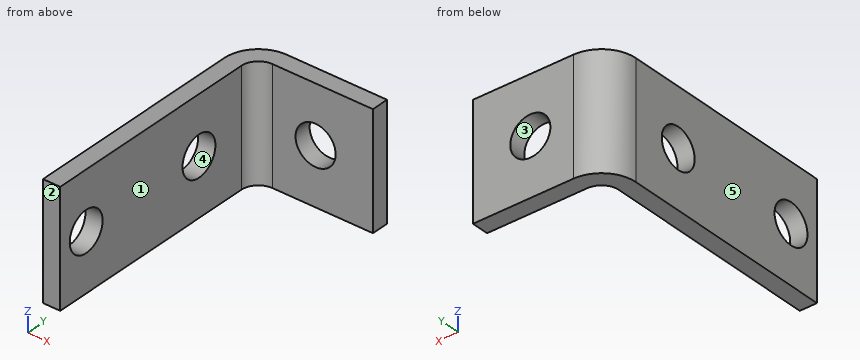
from build123d import *

# Parameters (mm, degrees)
BASE_FLANGE1_DEPTH             = 40
CUT_EXTRUDE1_DEPTH             = 109.350745652
F_14_0_14_DIAMETER_HOLE1_D     = 14
F_14_0_14_DIAMETER_HOLE1_DEPTH = 47
F_14_0_14_DIAMETER_HOLE2_D     = 14


# Sheet-metal steps are written as plain solids
with BuildPart() as part:
    # Sketch7 → Base-Flange1 (new body)
    with BuildSketch(Plane.XY):
        with BuildLine():
            Line((0, 0), (47, 0))
            Line((47, 0), (47, 89.055511246))
            Line((47, 89.055511246), (12, 89.055511246))
            ThreePointArc((12, 89.055511246), (3.514718626, 85.54079262), (0, 77.055511246))
            Line((0, 77.055511246), (0, 0))
        make_face()
    extrude(amount=-BASE_FLANGE1_DEPTH)

    # Sketch10 → Cut-Extrude1 (cut, through all)
    with BuildSketch(Plane(origin=(0, 0, -40), x_dir=(-1, 0, 0), z_dir=(0, 0, -1))):
        with BuildLine():
            Line((-12, 83.055511246), (-47, 83.055511246))
            Line((-47, 83.055511246), (-47, 0))
            Line((-47, 0), (-6, 0))
            Line((-6, 0), (-6, 77.055511246))
            ThreePointArc((-6, 77.055511246), (-7.757359313, 81.298151933), (-12, 83.055511246))
        make_face()
    extrude(amount=-CUT_EXTRUDE1_DEPTH, mode=Mode.SUBTRACT)

    # Ø14.0 (14) Diameter Hole1
    with Locations(Plane.ZY):
        with Locations((-20, 59.055511246), (-20, 11.055511246)):
            Hole(F_14_0_14_DIAMETER_HOLE1_D / 2, depth=F_14_0_14_DIAMETER_HOLE1_DEPTH)

    # Ø14.0 (14) Diameter Hole2 (through all)
    with Locations(Plane(origin=(0, 83.055511246, 0), x_dir=(-1, 0, 0), z_dir=(0, -1, 0))):
        with Locations((-27, 20)):
            Hole(F_14_0_14_DIAMETER_HOLE2_D / 2)


solid = part.part
Geometry: final body of the model. Coordinates: model frame, mm. Face numbers are marked on the shaded views. A direction names the side the tool comes from. Coordinates: 2 decimals unless noted, no trailing zeros. Order: outer loops, then holes, each group sorted by start corner. A loop starts at its lowest first (then second) coordinate and runs counter-clockwise, first axis right, second up.
(1) Draft query along X for the marked faces 3, 4 and 5. Return one class per face: pulls with the +X half, pulls with the -X half, needs draft (parallel to the pull), parting line crosses it, or undercut.
(2) First-contact query: pin 1 (22.5 mm diameter, centred on x = 27, z = -20, fed in from -Y); pin 2 (1.5 mm diameter, centred on x = 12, z = -6.5, fed in from -Y). Flat tips, straight axial feed; report the tip coordinate or a pass-through.
(3) Section query B-B (x = 27). Return the cut outline in (y, z), plus the area to 3 significant figures.
(4) Section query D-D (x = 16.5). Return the cut outline in (y, z), plus the area to 3 significant figures.
(5) Section query C-C (z = -11.5). Return the cut outline in (x, y), plus the area to 3 significant figures.
(6) Section query A-A (z = -20). Return the cut outline in (x, y), plus the area to 3 significant figures.
(7) Access query for the marked faces 1 and 2. Directions: +Z, -Z, +X, -X, +Y, -Y. A direction counts if a zero-diameter tool reaches every point of the face in a straight line with its end or side. Return the directions, or none.
(8) Material intervals for probe 1 along Y at (x, z) = (3, -20); probe 2 along Z at (x, y) = (27, 85); probe 3 along Y at (x, z) = (1, -20), sorted ascending.
Solution:
1. face 3: undercut
1. face 4: needs draft
1. face 5: pulls with the -X half
2. pin 1: stops at y = 83.06
2. pin 2: stops at y = 83.01
3. outline: (83.06, -40) - (89.06, -40) - (89.06, -27) - (83.06, -27) - close; (83.06, -13) - (89.06, -13) - (89.06, 0) - (83.06, 0) - close
3. area: 156 mm2
4. outline: (83.06, -40) - (89.06, -40) - (89.06, 0) - (83.06, 0) - close
4. area: 240 mm2
5. outline: (0, 0) - (6, 0) - (6, 77.06) arc R6 cw to (12, 83.06) - (47, 83.06) - (47, 89.06) - (12, 89.06) arc R12 ccw to (0, 77.06) - close
5. area: 757 mm2
6. outline: (0, 0) - (6, 0) - (6, 4.06) - (0, 4.06) - close; (0, 18.06) - (6, 18.06) - (6, 52.06) - (0, 52.06) - close; (0, 66.06) - (6, 66.06) - (6, 77.06) arc R6 cw to (12, 83.06) - (20, 83.06) - (20, 89.06) - (12, 89.06) arc R12 ccw to (0, 77.06) - close; (34, 83.06) - (47, 83.06) - (47, 89.06) - (34, 89.06) - close
6. area: 505 mm2
7. face 1: +Z, -Z, +X, -Y
7. face 2: +Z, -Z, +X, -X, -Y
8. probe 1: y = 0 to 4.06, 18.06 to 52.06, 66.06 to 84.99
8. probe 2: z = -40 to -27, -13 to 0
8. probe 3: y = 0 to 4.06, 18.06 to 52.06, 66.06 to 81.85
